The model under review builds one solid part; all positions refer to its coordinate system, in mm. Face numbers are marked on the shaded views. A direction names the side the tool comes from. Give positions to 0.01 mm unless a question says otherwise; leave off trailing zeros. Write each loop counter-clockwise with the first axis right and the second up, starting at its lowest first coordinate (ties: lowest second). Pieces come first, ordered by that corner, then holes. Notation, with made-up numbers: (-9.5, 68.5) - (39.5, 68.5) arc R31 cw to (39.5, 104.5) - close; hole circle Ø11 at (46.25, 69). An arc over 180 degrees is marked (long way). Write item = value, one per line.
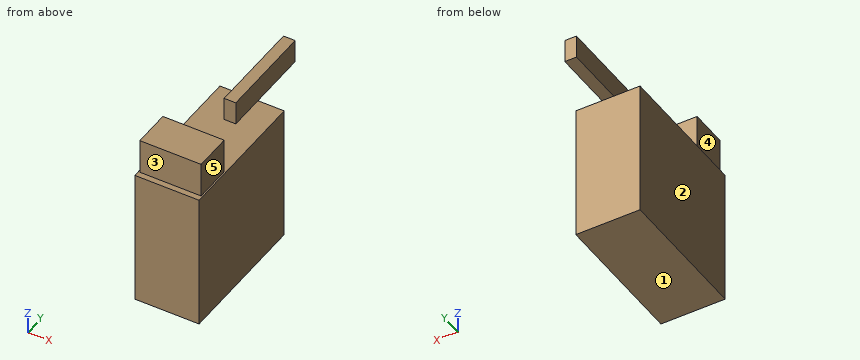
```python
from build123d import *

# Parameters (mm, degrees)
F0_W     = 533.4
F0_H     = 330.2
F1_DEPTH = 1193.8
F0_W_2   = 101.6
F0_H_2   = 533.4
F0_H_3   = 316.828786
F2_DEPTH = 1397
F3_DEPTH = 1498.6
F4_W     = 533.4
F4_H     = 1193.8
F5_DEPTH = 330.201


with BuildPart() as f1:
    # F0 (on Top) → F1 (new body)
    with BuildSketch(Plane.XY):
        Polygon((0, 1219.2), (0, 0), (558.8, 0), (558.8, 1219.2), (330.2, 1219.2), (330.2, 902.371214), (228.6, 902.371214), (228.6, 1219.2), align=None)
        with Locations((279.4, 215.9)):
            Rectangle(F0_W, F0_H, mode=Mode.SUBTRACT)
    extrude(amount=F1_DEPTH)

    # F0 (on Top) → F2 (join)
    with BuildSketch(Plane.XY):
        with Locations((279.4, 1485.9)):
            Rectangle(F0_W_2, F0_H_2)
        with Locations((279.4, 1060.785607)):
            Rectangle(F0_W_2, F0_H_3)
    extrude(amount=F2_DEPTH)

    # F0 (on Top) → F3 (join)
    with BuildSketch(Plane.XY):
        with Locations((279.4, 215.9)):
            Rectangle(F0_W, F0_H)
    extrude(amount=F3_DEPTH)

    # F4 (on face) → F5 (cut, through all)
    with BuildSketch(Plane(origin=(228.6, 0, 0), x_dir=(0, -1, 0), z_dir=(-1, 0, 0))):
        with Locations((-1485.9, 596.9)):
            Rectangle(F4_W, F4_H)
    extrude(amount=-F5_DEPTH, mode=Mode.SUBTRACT)


solid = f1.part
```
1. Take a section at C-C on x = 501.5. Give the boundary of the cut face in (y, z), and give its area (3 significant figures).
Findings below:
outline = (0, 0) - (1219.2, 0) - (1219.2, 1193.8) - (381, 1193.8) - (381, 1498.6) - (50.8, 1498.6) - (50.8, 1193.8) - (0, 1193.8) - close
area = 1,560,000 mm²
2. Take a section at D-D on z = 651.5. Give the boundary of the cut face in (x, y), and give its area (3 significant figures).
Findings below:
outline = (0, 0) - (558.8, 0) - (558.8, 1219.2) - (0, 1219.2) - close
area = 681,000 mm²
3. Machinability: for the marked faces 1, 2, 3, 4 and 5, which of the approach directions +Z, -Z, +X, -X, +Y, -Y give a long, thin tool a straight path to every point of the face, cutting with its end or side? Answer none if there is none.
Findings below:
face_1 = -Z, +X, -X, +Y, -Y
face_2 = +Z, -Z, -X, +Y, -Y
face_3 = +Z, +X, -X, -Y
face_4 = +Z, -X, +Y, -Y
face_5 = +Z, +X, +Y, -Y
4. Insertion check: P1, Ø1, axis at x = 352, z = 281, coming from the +Y side. The pin has a flat end and moves straight along its axis. Give the tip position at first contact, or say it passes through.
Findings below:
P1 = 1219.2
5. Take a section at B-B on y = 1080. Give the boundary of the cut face in (x, z), and give its area (3 significant figures).
Findings below:
outline = (0, 0) - (558.8, 0) - (558.8, 1193.8) - (330.2, 1193.8) - (330.2, 1397) - (228.6, 1397) - (228.6, 1193.8) - (0, 1193.8) - close
area = 688,000 mm²
6. For line 1 (Z direction, x = 119, y = 870); line 2 (Y direction, x = 344.5, z = 639.5); line 3 (X direction, y = 910.5, z = 1348), list the stretches that pass through material, from the lowest coordinate up. Write a range as from..to.
Findings below:
line_1 = 0..1193.8
line_2 = 0..1219.2
line_3 = 228.6..330.2
7. Take a section at A-A on z = 1271. Give the boundary of the cut face in (x, y).
Findings below:
outline = (12.7, 50.8) - (546.1, 50.8) - (546.1, 381) - (12.7, 381) - close; (228.6, 902.37) - (330.2, 902.37) - (330.2, 1752.6) - (228.6, 1752.6) - close
